Can you work these out from the model? Positions are in its coordinate system, mm. A direction names the side the tool comes from. Round coordinates to 2 decimals unless told otherwise and drop trailing zeros. Order: outer loops, then holes, each group sorted by start corner. A loop starts at its lowest first (then second) coordinate and runs counter-clockwise, first axis right, second up.
Autodesk Inventor part; units mm, degrees
ref_plane "Work Plane1" through (0, 5.825, 0) normal (0, 1, 0) x (-1, 0, 0)
ref_plane "YZ Plane" through (0, 0, 0) normal (1, 0, 0) x (0, 1, 0)
ref_plane "XZ Plane" through (0, 0, 0) normal (0, 1, 0) x (-1, 0, 0)
sketch "Sketch1" plane through (0, 0, 0) normal (0, 0, 1) x (1, 0, 0)
  circle A0 centre (0, 0) radius 3.825
  circle A1 centre (0, 0) radius 5.825
  dimension "d0" = 7.65
  dimension "d1" = 2
extrude "Extrusion1" add sketch "Sketch1" along normal blind 10
sketch "Sketch2" plane through (0, 0, 10) normal (0, 0, 1) x (1, 0, 0)
  circle A0 centre (0, 0) radius 4
  dimension "d4" = 8
extrude "Extrusion2" add sketch "Sketch2" along normal mid plane 6
move faces "Move1" translate (0, 0, 2.5) faces at (0.7574, 1.0973, 13)
sketch "Sketch3" plane through (0, 0, 0) normal (0, 0, -1) x (-1, 0, 0)
  line L0 (0, 0) -> (0, 5.825)
  circle A0 centre (0, 0) radius 5.825
ref_plane "Work Plane1" through (0, 5.825, 0) normal (0, 1, 0) x (-1, 0, 0)
sketch "Sketch4" plane through (0, 5.825, 0) normal (0, 1, 0) x (-1, 0, 0)
  circle A0 centre (0, 4.3) radius 1.5
  point P0 (0, 0)
  dimension "d10" = 3
  dimension "d11" = 4.3
extrude "Extrusion3" cut sketch "Sketch4" against normal through all
properties part number "shaft_extension2"
(1) I want a section at B-B, the plane x = 0. List the corners of the cut face in (y, z) for me (3 decimals), plus the area to 4 significant figures.
(2) I'm going to push flat-ended pins straight in: pin 1 Ø3 at (x, z) = (0.5, 2) entering from -Y (3 decimals); pin 2 Ø3 at (x, z) = (-1.5, 13) entering from -Y; pin 3 Ø2.5 at (x, y) = (-1.5, -2) entering from -Z. Where does each tip first touch, or does it pass through?
(3) On a 3-axis mill with a long thin cutter (end or side, diameter ignored), from which of +Z, -Z, +X, -X, +Y, -Y can I reach the whole of each face in a straight line? I mean faces 4 (the face through (1.2, 4, 10)), 5 (the face through (1, -4, 0)), 6 (the face through (0, 0, 7)). Say none if no direction works.
(4) I want a section at A-A, the plane z = 4.3. List the corners of the cut face in (x, y) for me (3 decimals).
(5) Please list where these lines run through material, in increasing order: probe 1 along Y at (x, z) = (0, 1.5) (3 decimals); probe 2 along Z at (x, y) = (0, 4.05); probe 3 along Z at (x, y) = (5, -2).
(6) I want a section at C-C, the plane y = 0. List the corners of the cut face in (x, z) for me (3 decimals).
(7) If we mould it in two halves opening along Y, with no side actions, what happens to faces 1 (the face through (-0.867, 3.905, 12.712)), 2 (the face through (3.533, 1.465, 3.451)), 3 (the face through (0, 0, 15.5))? For each: pulls with the +Y half, pulls with the -Y half, needs draft (parallel to the pull), parting line crosses it, or undercut.
(8) I want a section at D-D, the plane x = -2.25. List the corners of the cut face in (y, z) for me, plus the area to 3 significant figures.
Ans:
1. outline: (-5.825, 0) - (-3.825, 0) - (-3.825, 2.8) - (-5.825, 2.8) - close; (-5.825, 5.8) - (-3.825, 5.8) - (-3.825, 7) - (3.825, 7) - (3.825, 5.8) - (5.825, 5.8) - (5.825, 10) - (4, 10) - (4, 15.5) - (-4, 15.5) - (-4, 10) - (-5.825, 10) - close; (3.825, 0) - (5.825, 0) - (5.825, 2.8) - (3.825, 2.8) - close
1. area: 94.95 mm2
2. pin 1: stops at y = -5.825
2. pin 2: stops at y = -4
2. pin 3: stops at z = 7
3. face 4: +Z
3. face 5: -Z, +X, -X, +Y, -Y
3. face 6: -Z
4. outline: (-1.5, -5.629) - (-1.5, -3.519) arc R3.825 cw to (-1.5, 3.519) - (-1.5, 5.629) arc R5.825 ccw to start; (1.5, -5.629) arc R5.825 ccw to (1.5, 5.629) - (1.5, 3.519) arc R3.825 cw to (1.5, -3.519) - close
5. probe 1: y = -5.825 to -3.825, 3.825 to 5.825
5. probe 2: z = 0 to 2.8, 5.8 to 10
5. probe 3: z = 0 to 10
6. outline: (-5.825, 0) - (-3.825, 0) - (-3.825, 7) - (3.825, 7) - (3.825, 0) - (5.825, 0) - (5.825, 10) - (4, 10) - (4, 15.5) - (-4, 15.5) - (-4, 10) - (-5.825, 10) - close
7. face 1: parting line crosses it
7. face 2: undercut
7. face 3: needs draft
8. outline: (-5.37, 0) - (-3.09, 0) - (-3.09, 7) - (3.09, 7) - (3.09, 0) - (5.37, 0) - (5.37, 10) - (3.31, 10) - (3.31, 15.5) - (-3.31, 15.5) - (-3.31, 10) - (-5.37, 10) - close
8. area: 101 mm2
